Autodesk Inventor part; units mm, degrees
ref_plane "montageblocke_XY" through (0, -8.75, 3.5) normal (0, 0, 1) x (1, 0, 0)
ref_plane "montageblocke_YZ" through (0, -8.75, 3.5) normal (1, 0, 0) x (0, 1, 0)
ref_plane "montageblocke_ZX" through (0, -8.75, 3.5) normal (0, 1, 0) x (0, 0, 1)
sketch "Sketch_1" plane through (0, 0, 0) normal (0, 1, 0) x (-1, 0, 0)
  line L0 (5.5, 0) -> (-6.3, 0)
  line L1 (-6.3, 0) -> (-5.1732, -21.5)
  line L2 (-5.1732, -21.5) -> (4.3732, -21.5)
  line L3 (4.3732, -21.5) -> (5.5, 0)
extrude "Extrusion1" add sketch "Sketch_1" along normal mid plane 26.8
sketch "Sketch_2" plane through (0, 0, 0) normal (1, 0, 0) x (0, 1, 0)
  line L0 (13.4, 0) -> (12.2732, -21.5)
  line L1 (12.2732, -21.5) -> (-12.2732, -21.5)
  line L2 (-12.2732, -21.5) -> (-13.4, 0)
  line L3 (-13.4, 0) -> (-15, 0)
  line L4 (-15, 0) -> (-15, -25)
  line L5 (-15, -25) -> (15, -25)
  line L6 (15, -25) -> (15, 0)
  line L7 (15, 0) -> (13.4, 0)
extrude "Extrusion2" cut sketch "Sketch_2" along normal mid plane 13
sketch "Sketch_3" plane through (-7, 0, 0) normal (1, 0, 0) x (0, 0, -1)
  line L0 (0, -7.9) -> (18.5, -7.9)
  line L1 (18.5, -7.9) -> (21.5, -6.1679)
  line L2 (21.5, -6.1679) -> (21.5, 6.1679)
  line L3 (21.5, 6.1679) -> (18.5, 7.9)
  line L4 (18.5, 7.9) -> (0, 7.9)
  line L5 (0, 7.9) -> (0, -7.9)
extrude "Extrusion3" add sketch "Sketch_3" along normal blind 13.3
sketch "Sketch_4" plane through (0, 0, 0) normal (0, 1, 0) x (-1, 0, 0)
  line L0 (7, 0) -> (7, 3)
  arc A0 (7, 3) -> (6.5, 3.5) centre (6.5, 3) ccw
  line L1 (6.5, 3.5) -> (-4.8, 3.5)
  arc A1 (-4.8, 3.5) -> (-7.8, 0.5) centre (-4.8, 0.5) ccw
  arc A2 (-7.8, 0.5) -> (-7.3, 0) centre (-7.3, 0.5) ccw
  line L2 (-7.3, 0) -> (7, 0)
extrude "Extrusion4" add sketch "Sketch_4" along normal mid plane 30
sketch "Sketch5" plane through (-6.5, 15, 3.5) normal (0, 0, 1) x (1, 0, 0)
  point P0 (6.5, -6.25)
hole "Drilling 1" at (0, 8.75, 3.5) direction (0, 0, -1) diameter 3.1 depth 11.2 tip angle 120 counterbore diameter 4 counterbore depth 0.7
sketch "Sketch6" plane through (-6.5, 15, 3.5) normal (0, 0, 1) x (1, 0, 0)
  point P0 (6.5, -23.75)
hole "Drilling 2" at (0, -8.75, 3.5) direction (0, 0, -1) diameter 3.1 depth 11.2 tip angle 120 counterbore diameter 4 counterbore depth 0.7
sketch "Sketch7" plane through (5.1732, 12.2732, -21.5) normal (0, 0, -1) x (-1, 0, 0)
  point P0 (5.1732, -6.0232)
hole "Drilling 3" at (0, 6.25, -21.5) direction (0, 0, 1) diameter 3.1 depth 10 tip angle 120 counterbore diameter 4 counterbore depth 1.5
sketch "Sketch8" plane through (5.1732, 12.2732, -21.5) normal (0, 0, -1) x (-1, 0, 0)
  point P0 (5.1732, -18.5232)
hole "Drilling 4" at (0, -6.25, -21.5) direction (0, 0, 1) diameter 3.1 depth 10 tip angle 120 counterbore diameter 4 counterbore depth 1.5
sketch "Sketch9" plane through (-7, 0, 0) normal (-1, 0, 0) x (0, 0, 1)
  point P0 (-15, 0)
hole "Drilling 5" at (-7, 0, -15) direction (1, 0, 0) diameter 3.1 depth 11 tip angle 120 counterbore diameter 4 counterbore depth 1.5
ref_plane "montageblocke_XY" through (0, -8.75, 3.5) normal (0, 0, 1) x (1, 0, 0)
ref_plane "montageblocke_YZ" through (0, -8.75, 3.5) normal (1, 0, 0) x (0, 1, 0)
ref_plane "montageblocke_ZX" through (0, -8.75, 3.5) normal (0, 1, 0) x (0, 0, 1)
ref_plane "montageblocke_2_XY" through (0, 8.75, 3.5) normal (0, 0, 1) x (1, 0, 0)
ref_plane "montageblocke_2_YZ" through (0, 8.75, 3.5) normal (1, 0, 0) x (0, 1, 0)
ref_plane "montageblocke_2_ZX" through (0, 8.75, 3.5) normal (0, 1, 0) x (0, 0, 1)
properties part number "1XXX.500_Montageblocke"
Design review of the part built by this model. Coordinates are the model's own, in mm. A direction names the side the tool comes from. Round coordinates to 2 decimals unless told otherwise and drop trailing zeros. Loops run counter-clockwise (first coordinate to the right, second up) from the corner with the lowest first, then second, coordinate; pieces in that order, holes last. Notation, with made-up numbers: (65, 61.5) - (111, 61.5) arc R17 ccw to (111, 89.5) - close; hole circle Ø3 at (29.25, 64). An arc over 180 degrees is marked (long way). One line per question, with ' | ' between items.
1. For faces 4 (the face through (-5.705, 7.022, -20.021)), 5 (the face through (1.217, 10.337, 3.145)), 6 (the face through (5.744, -10.638, -10.6)), list the 3-axis set-ups (+Z, -Z, +X, -X, +Y, -Y) from which the entire face can be reached by the end or side of a thin tool; tool diameter is ignored.
Results are:
face 4: -Z, -X, +Y | face 5: +Z | face 6: -Z, +X, -Y
2. For L1, parallel to Y at x = 0, z = 3.3; L2, parallel to X at y = -6.25, z = -15; L3, parallel to Y at x = 0, z = -2, list the stretches that pass through material, from the lowest coordinate up. Write a range as [from, to].
Results are:
L1: y = [-15, -10.75], [-6.75, 6.75], [10.75, 15] | L2: x = [-7, -1.55], [1.55, 6.3] | L3: y = [-13.3, -10.3], [-7.2, 7.2], [10.3, 13.3]
3. Draft analysis for pull direction Z (two halves, no side actions). For faces 1 (the face through (4.74, 0.01, -15.27)), 2 (the face through (0, 0, -21.5)), 3 (the face through (-6, 7.9, -9)), state which applies: released by +Z, released by -Z, zero draft, split by the parting line, or undercut.
Results are:
face 1: undercut | face 2: released by -Z | face 3: zero draft
4. We need section C-C, the plane z = 1. State the section outline as (x, y) points, and give its area (3 significant figures).
Results are:
outline: (-7, -15) - (7.76, -15) - (7.76, 15) - (-7, 15) - close; hole circle Ø3.1 at (0, -8.75); hole circle Ø3.1 at (0, 8.75) | area: 428 mm²
5. We need section B-B, the plane x = -6. State the section outline as (y, z) points, and give its area (3 significant figures).
Results are:
outline: (-15, 0) - (-7.9, 0) - (-7.9, -18.5) - (-6.17, -21.5) - (6.17, -21.5) - (7.9, -18.5) - (7.9, 0) - (15, 0) - (15, 3.5) - (-15, 3.5) - close; hole circle Ø4 at (0, -15) | area: 427 mm²
6. Clearance check with flat-ended pins moving along their axes: P1, Ø5, axis at x = 0, y = 8.75, coming from the +Z side; P2, Ø1, axis at y = -8.5, z = -6.5, coming from the -X side; P3, Ø2, axis at x = -0.5, z = -5, coming from the +Y side; P4, Ø0.8, axis at x = 6, z = -6.5, coming from the +Y side. State where each tip first meets the part, or that it passes through.
Results are:
P1: stops at z = 3.5 | P2: stops at x = -5.19 | P3: stops at y = 13.19 | P4: stops at y = 13.08
7. We need section A-A, the plane x = -2.5. State the section outline as (y, z) points, and give its area (3 significant figures).
Results are:
outline: (-15, 0) - (-13.4, 0) - (-12.27, -21.5) - (12.27, -21.5) - (13.4, 0) - (15, 0) - (15, 3.5) - (-15, 3.5) - close; hole circle Ø3.1 at (0, -15) | area: 649 mm²
